Verification items for the finished model (mm, model axes). A direction names the side the tool comes from. Round coordinates to 2 decimals unless told otherwise and drop trailing zeros. Order: outer loops, then holes, each group sorted by start corner. A loop starts at its lowest first (then second) coordinate and runs counter-clockwise, first axis right, second up. Notation, with made-up numbers: (55, 11.5) -> (70, 11.5) arc R11 cw to (70, 22.5) -> close; hole circle Ø2 at (-40, 88). An arc over 180 degrees is marked (long way). Put each result on its own line as item: value.
```python
from build123d import *

# Parameters (mm, degrees)
F0_R     = 1.5
F1_DEPTH = 1.5
F2_R     = 0.5
F3_R     = 1
F4_DEPTH = 15


with BuildPart() as f1:
    # F0 (on Front) → F1 (new body)
    with BuildSketch(Plane.XZ):
        Circle(F0_R)
    extrude(amount=F1_DEPTH)

    # F2
    f2_edges = [f1.edges().sort_by_distance(p)[0] for p in [
        (-1.5, -1.5, 0),
    ]]
    fillet(f2_edges, radius=F2_R)

    # F3 (on face) → F4 (join)
    with BuildSketch(Plane(origin=(0, 0, 0), x_dir=(-1, 0, 0), z_dir=(0, 1, 0))):
        Circle(F3_R)
    extrude(amount=F4_DEPTH)


solid = f1.part
```
Item 1: Tool access check on faces 1 (the face through (0, 7, -1)), 2 (the face through (-1.5, -0.49, 0.07)). Record the directions out of +Z, -Z, +X, -X, +Y, -Y that give a thin tool (end or side, any length) a straight path to the whole face; none if there is none.
Geometry check:
face 1: +Y
face 2: +Y, -Y
Item 2: Material ranges on line 1 along Z through (x, y) = (0.35, 13); line 2 along Z through (x, y) = (-0.65, 10.25); line 3 along X through (y, z) = (10, -0.9), recorded low to high.
Geometry check:
line 1: -0.94 to 0.94
line 2: -0.76 to 0.76
line 3: -0.44 to 0.44
Item 3: Sectioned sample at A-A, the plane z = 0. Record the boundary of the cut face in (x, y), then the cut area to 3 significant figures.
Geometry check:
outline: (-1.5, -1) arc R0.5 ccw to (-1, -1.5) -> (1, -1.5) arc R0.5 ccw to (1.5, -1) -> (1.5, 0) -> (1, 0) -> (1, 15) -> (-1, 15) -> (-1, 0) -> (-1.5, 0) -> close
area: 34.4 mm2
Item 4: Sectioned sample at B-B, the plane x = 0. Record the boundary of the cut face in (y, z).
Geometry check:
outline: (-1.5, -1) arc R0.5 ccw to (-1, -1.5) -> (0, -1.5) -> (0, -1) -> (15, -1) -> (15, 1) -> (0, 1) -> (0, 1.5) -> (-1, 1.5) arc R0.5 ccw to (-1.5, 1) -> close
Item 5: Sectioned sample at C-C, the plane y = 5.75. Record the boundary of the cut face in (x, z).
Geometry check:
outline: circle Ø2 at (0, 0)
